from build123d import *

# Parameters (mm, degrees)
F0_R     = 89
F0_R_2   = 28
F1_DEPTH = 1
F2_D     = 10.5
F3_D     = 30
F4_D     = 3
F6_D     = 3


with BuildPart() as f1:
    # F0 (on Front) → F1 (new body)
    with BuildSketch(Plane.XZ):
        Circle(F0_R)
        Circle(F0_R_2, mode=Mode.SUBTRACT)
    extrude(amount=-F1_DEPTH)

    # F2 (through all)
    with Locations(Plane.XZ):
        with Locations((-54.2102163981, -17.6139841623), (54.2102163981, -17.6139841623)):
            Hole(F2_D / 2)

    # F3 (through all)
    with Locations(Plane.XZ):
        with Locations((-54.2102264595, 17.6139531965), (0, 57), (54.2102264595, 17.6139531965), (33.5032664595, -46.1143268035), (-33.5032664595, -46.1143268035)):
            Hole(F3_D / 2)

    # F4 (through all)
    with Locations(Plane.XZ):
        with Locations((-30.4338113457, 9.8885351278), (0, 32), (30.4338113457, 9.8885351278), (18.8088513457, -25.8887448722), (-18.8088513457, -25.8887448722)):
            Hole(F4_D / 2)

    # F6 (through all)
    with Locations(Plane.XZ):
        with Locations((-60.811183182, 60.811183182), (0, 86), (60.811183182, 60.811183182), (86, 0), (60.811183182, -60.811183182), (0, -86), (-60.811183182, -60.811183182), (-86, 0)):
            Hole(F6_D / 2)


solid = f1.part
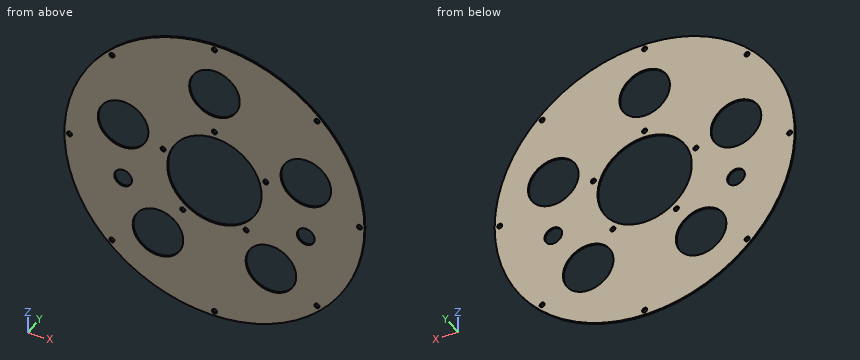
Source: CAD feature listing. Evaluate the final solid. Frame: model axes, mm. Give positions to 0.01 mm unless a question says otherwise; leave off trailing zeros. Write each loop counter-clockwise with the first axis right and the second up, starting at its lowest first coordinate (ties: lowest second). Pieces come first, ordered by that corner, then holes. Notation, with made-up numbers: M -36,-13 L -27,-13 A13 ccw -27,-5 Z; hole C 55.5,71.25 d9. An arc over 180 degrees is marked long. Answer as a JSON object with one key per item and string values.
Q1. Ray query, line 1 along X through (y, z) = (0.4, 19); line 2 along X through (y, z) = (0.8, -50.5); line 3 along X through (y, z) = (0.2, -25). Return the intervals inside material, ascending.
Geometry check:
{"line 1": "x = -86.95 to -69.15, -39.27 to -20.57, 20.57 to 39.27, 69.15 to 86.95", "line 2": "x = -73.29 to -47.85, -19.16 to 19.16, 47.85 to 73.29", "line 3": "x = -85.42 to -20.02, -17.6 to -12.61, 12.61 to 17.6, 20.02 to 85.42"}
Q2. Cut plane C-C, the plane y = 0.35. Count the separate pieces of the cut face and the enclosed holes in it, then the cut area to 3 significant figures.
Geometry check:
{"separate pieces": "1", "enclosed holes": "21", "area": "18,600 mm^2"}
Q3. Cut plane B-B, the plane z = 46.5. Return the cut outline in (x, y), then the cut area to 3 significant figures.
Geometry check:
{"outline": "M -75.89,0 L -10.71,0 L -10.71,1 L -75.89,1 Z; M 10.71,0 L 75.89,0 L 75.89,1 L 10.71,1 Z", "area": "130 mm^2"}
Q4. Contact query for flat-ended pins moving along their axis: P1, Ø10, axis at x = 33, z = -19, coming from the -Y side; P2, Ø2.5, axis at x = 0, z = 32, coming from the +Y side. Output: stop coordinate, or through.
Geometry check:
{"P1": "stops at y = 0", "P2": "passes through"}
Q5. Cut plane D-D, the plane x = -23. Return the cut outline in (y, z), then the cut area to 3 significant figures.
Geometry check:
{"outline": "M 0,-85.98 L 1,-85.98 L 1,-56.82 L 0,-56.82 Z; M 0,-35.41 L 1,-35.41 L 1,-15.97 L 0,-15.97 Z; M 0,15.97 L 1,15.97 L 1,85.98 L 0,85.98 Z", "area": "119 mm^2"}
Q6. Cut plane A-A, the plane x = 55.5. Return the cut outline in (y, z).
Geometry check:
{"outline": "M 0,-69.58 L 1,-69.58 L 1,-22.7 L 0,-22.7 Z; M 0,-12.52 L 1,-12.52 L 1,2.67 L 0,2.67 Z; M 0,32.56 L 1,32.56 L 1,69.58 L 0,69.58 Z"}
